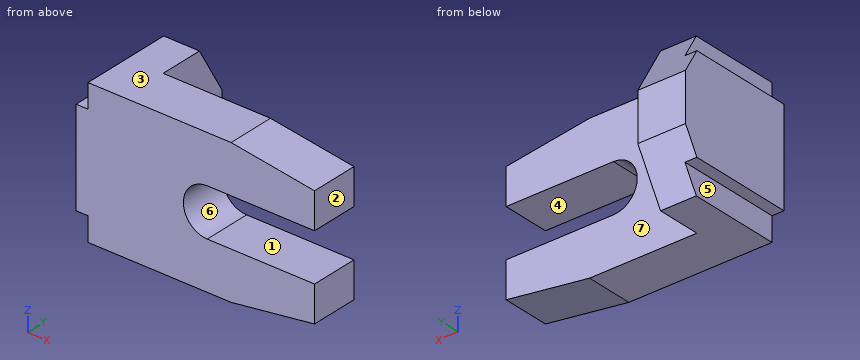
```python
from build123d import *

# Parameters (mm, degrees)
EXTRUDE_1_DEPTH     = 25.4
EXTRUDE_2_DEPTH     = 63.5
CUT_EXTRUDE_1_DEPTH = 63.5


with BuildPart() as part:
    # 草图2 → 凸台-拉伸1 (new body)
    with BuildSketch(Plane(origin=(0, 0, 0), x_dir=(1, 0, 0), z_dir=(0, 1, 0))):
        with BuildLine():
            Line((0, 0), (0, 38.1))
            Line((0, 38.1), (57.15, 38.1))
            Line((57.15, 38.1), (101.6, 31.75))
            Line((101.6, 31.75), (101.6, 12.7))
            Line((101.6, 12.7), (44.45, 12.7))
            ThreePointArc((44.45, 12.7), (31.75, 0), (44.45, -12.7))
            Line((44.45, -12.7), (101.6, -12.7))
            Line((101.6, -12.7), (101.6, -31.75))
            Line((101.6, -31.75), (57.15, -38.1))
            Line((57.15, -38.1), (0, -38.1))
            Line((0, -38.1), (0, 0))
        make_face()
    extrude(amount=EXTRUDE_1_DEPTH)

    # 草图4 → 凸台-拉伸2 (add)
    with BuildSketch(Plane(origin=(0, 0, 0), x_dir=(-1, 0, 0), z_dir=(0, -1, 0))):
        Polygon((0, 38.1), (0, -38.1), (19.05, -38.1), (19.05, -25.4), (25.4, -25.4), (25.4, 25.4), (19.05, 25.4), (19.05, 38.1), align=None)
    extrude(amount=-EXTRUDE_2_DEPTH)

    # 草图5 → 切除-拉伸1 (cut)
    with BuildSketch(Plane(origin=(0, 0, 0), x_dir=(0, 0, -1), z_dir=(1, 0, 0))):
        Polygon((-38.1, 63.5), (-38.1, 48.835303163), (-12.7, 63.5), align=None)
        Polygon((38.1, 63.5), (12.7, 63.5), (38.1, 48.835303163), align=None)
    extrude(amount=-CUT_EXTRUDE_1_DEPTH, mode=Mode.SUBTRACT)


solid = part.part
```
Design review of the part built by this model. Coordinates are the model's own, in mm. Face numbers are marked on the shaded views. A direction names the side the tool comes from. Give positions to 0.01 mm unless a question says otherwise; leave off trailing zeros. Order: outer loops, then holes, each group sorted by start corner. A loop starts at its lowest first (then second) coordinate and runs counter-clockwise, first axis right, second up. Notation, with made-up numbers: (30, 43) - (39, 43) arc R8 cw to (39, 58) - close; hole circle Ø11 at (81, 12). An arc over 180 degrees is marked (long way). Use a Markdown table: item, result. Add a question column.
(1) Add section D-D on x = -10. Give the boundary of the cut face in (y, z), then the cut area to 3 significant figures.
(2) Mouldability with a two-part tool opening along Z and no side actions: class the marked faces 1, 2, 3 and 4 as +Z half, -Z half, draft (parallel to the pull), parting line (faces both ways), or undercut.
(3) Wall thickness on probe 1 along Z at (x, y) = (51, 7.5); probe 2 along X at (y, z) = (39, -10); probe 3 along Y at (x, z) = (17, -14): over which ranges is each line inside the solid? List them lowest first. Write a range as [from, to].
(4) Add section A-A on y = 28.5. Give the boundary of the cut face in (x, z), then the cut area to 3 significant figures.
(5) Add section B-B on x = 38. Give the boundary of the cut face in (y, z).
(6) Machinability: for the marked faces 5, 6 and 7, which of the approach directions +Z, -Z, +X, -X, +Y, -Y give a long, thin tool a straight path to every point of the face, cutting with its end or side? Answer none if there is none.
(7) Add section C-C on z = 0. Give the boundary of the cut face in (x, y), then the cut area to 3 significant figures.
(8) Clearance check with flat-ended pins moving along their axes: P1, Ø3, axis at y = 10, z = 6, coming from the +X side; P2, Ø1.9, axis at x = -22.5, y = 41, coming from the +Z side; P3, Ø8, axis at y = 37.5, z = 2.5, coming from the +X side. State where each tip first meets the part, or that it passes through.
Report:
| question | item | result |
|---|---|---|
| 1 | outline | (0, -38.1) - (48.84, -38.1) - (63.5, -12.7) - (63.5, 12.7) - (48.84, 38.1) - (0, 38.1) - close |
| 1 | area | 4,470 mm² |
| 2 | face 1 | undercut |
| 2 | face 2 | draft |
| 2 | face 3 | +Z half |
| 2 | face 4 | undercut |
| 3 | probe 1 | z = [-38.1, -12.7], [12.7, 38.1] |
| 3 | probe 2 | x = [-25.4, 0] |
| 3 | probe 3 | y = [0, 25.4] |
| 4 | outline | (-25.4, -25.4) - (-19.05, -25.4) - (-19.05, -38.1) - (0, -38.1) - (0, 38.1) - (-19.05, 38.1) - (-19.05, 25.4) - (-25.4, 25.4) - close |
| 4 | area | 1,770 mm² |
| 5 | outline | (0, -38.1) - (25.4, -38.1) - (25.4, -10.94) - (0, -10.94) - close; (0, 10.94) - (25.4, 10.94) - (25.4, 38.1) - (0, 38.1) - close |
| 6 | face 5 | -Z, -X, +Y, -Y |
| 6 | face 6 | +X, +Y, -Y |
| 6 | face 7 | +Z, -Z, +X, +Y |
| 7 | outline | (-25.4, 0) - (31.75, 0) - (31.75, 25.4) - (0, 25.4) - (0, 63.5) - (-25.4, 63.5) - close |
| 7 | area | 2,420 mm² |
| 8 | P1 | stops at x = 34.2 |
| 8 | P2 | stops at z = 25.4 |
| 8 | P3 | stops at x = 0 |
